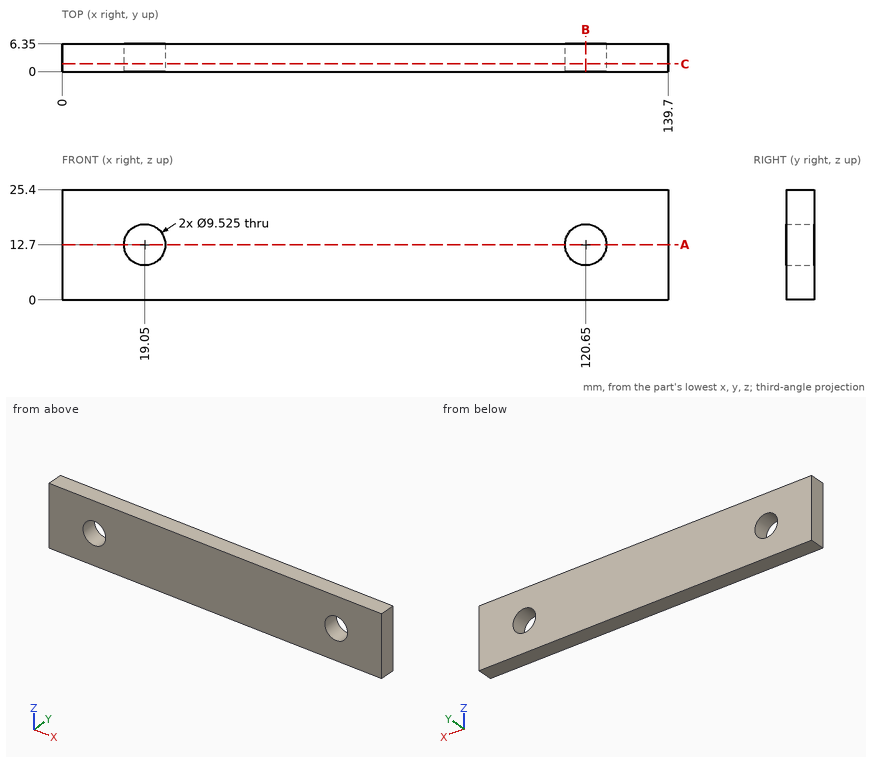
Job drawing, mm, ordinate dimensions from the low corner. One solid piece. Coordinates: 2 decimals unless noted, no trailing zeros. Loops run counter-clockwise (first coordinate to the right, second up) from the corner with the lowest first, then second, coordinate; pieces in that order, holes last. Notation, with made-up numbers: (30, 7) - (88, 7) arc R8 ccw to (88, 19) - close; hole circle Ø7 at (-38, -10.5). An arc over 180 degrees is marked (long way). Write item = value, one per line. Start each with the question number.
Q1. Cut at C-C, the plane y = 1.75. Give the number of separate pieces and of enclosed holes in the cut face, then the cut area to 3 significant figures.
Q2. Drill centre lines: L1, parallel to X at y = 5, z = 12.7; L2, parallel to X at y = 5.25, z = 10.75; L3, parallel to Z at x = 120.65, y = 4. Where is each one in solid material? Low to high.
Q3. Cut at A-A, the plane z = 12.7. List the corners of the cut face in (x, y), then the cut area to 3 significant figures.
Q4. Cut at B-B, the plane x = 120.65. List the corners of the cut face in (y, z).
Q5. Flat gauge pin, fed straight in: pin 1 Ø7.5 at (x, z) = (120.65, 12.7) entering from +Y. Where does the tip first touch, or does it go through?
Computed:
q1.separate_pieces = 1
q1.enclosed_holes = 2
q1.area = 3,410 mm²
q2.L1 = 0 to 14.29, 23.81 to 115.89, 125.41 to 139.7
q2.L2 = 0 to 14.71, 23.39 to 116.31, 124.99 to 139.7
q2.L3 = 0 to 7.94, 17.46 to 25.4
q3.outline = (0, 0) - (14.29, 0) - (14.29, 6.35) - (0, 6.35) - close; (23.81, 0) - (115.89, 0) - (115.89, 6.35) - (23.81, 6.35) - close; (125.41, 0) - (139.7, 0) - (139.7, 6.35) - (125.41, 6.35) - close
q3.area = 766 mm²
q4.outline = (0, 0) - (6.35, 0) - (6.35, 7.94) - (0, 7.94) - close; (0, 17.46) - (6.35, 17.46) - (6.35, 25.4) - (0, 25.4) - close
q5.pin_1 = through
